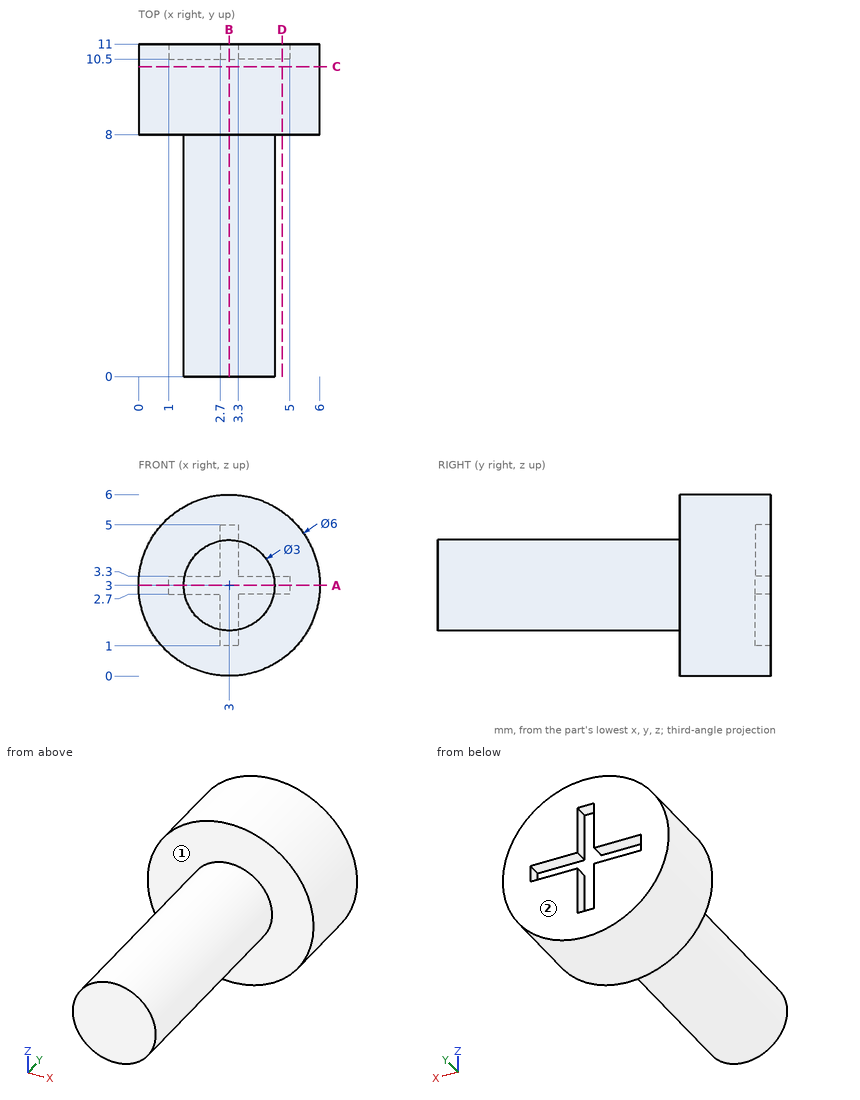
Here's the drawing with two shaded views (mm, measured from the low corner). I have some questions. A direction names the side the tool comes from. Give positions to 0.01 mm unless a question says otherwise; leave off trailing zeros. Write each loop counter-clockwise with the first axis right and the second up, starting at its lowest first coordinate (ties: lowest second). Pieces come first, ordered by that corner, then holes. Notation, with made-up numbers: (-7, -12) - (48, -12) arc R17 cw to (48, 1) - close; hole circle Ø8 at (68, 13.5). An arc over 180 degrees is marked (long way). One line per item, written item: value. Start each with the question number.
Item 1: Imagine slicing it at D-D, the plane x = 4.75. List the corners of the cut face in (y, z) for me.
Item 2: Please list where these lines run through material, in increasing order: line 1 (Y direction, x = 4.85, z = 1.85); line 2 (Y direction, x = 4.9, z = 3.2); line 3 (X direction, y = 7, z = 2.9). Write a range as from..to.
Item 3: Which directions (+Z, -Z, +X, -X, +Y, -Y) give clear straight access to the entire face, cutting with the end or side of a thin tool? Please do the marked faces 1 and 2.
Item 4: I'm going to push flat-ended pins straight in: pin 1 (3 mm diameter, centred on x = 0.5, y = 8.5, fed in from +Z); pin 2 (3 mm diameter, centred on x = 1.5, y = 3, fed in from +Z); pin 3 (0.6 mm diameter, centred on y = 10.5, z = 4, fed in from -X). Where does each tip first touch, or does it pass through?
Item 5: Imagine slicing it at B-B, the plane x = 3. List the corners of the cut face in (y, z) for me.
Item 6: Imagine slicing it at C-C, the plane y = 10.25. List the corners of the cut face in (x, z) for me.
Item 7: Imagine slicing it at A-A, the plane z = 3. List the corners of the cut face in (x, y) for me.
Geometry says:
1. outline: (8, 0.56) - (11, 0.56) - (11, 2.7) - (10.5, 2.7) - (10.5, 3.3) - (11, 3.3) - (11, 5.44) - (8, 5.44) - close
2. line 1: 8..11
2. line 2: 8..10.5
2. line 3: 1.5..4.5
3. face 1: -Y
3. face 2: +Z, -Z, +X, -X, +Y
4. pin 1: z = 5.83
4. pin 2: z = 4.5
4. pin 3: x = 0.08
5. outline: (0, 1.5) - (8, 1.5) - (8, 0) - (11, 0) - (11, 1) - (10.5, 1) - (10.5, 5) - (11, 5) - (11, 6) - (8, 6) - (8, 4.5) - (0, 4.5) - close
6. outline: circle Ø6 at (3, 3)
7. outline: (0, 8) - (1.5, 8) - (1.5, 0) - (4.5, 0) - (4.5, 8) - (6, 8) - (6, 11) - (5, 11) - (5, 10.5) - (1, 10.5) - (1, 11) - (0, 11) - close
